Part print with two shaded views. Sizes in mm from the minimum x, y, z corner. Round coordinates to 2 decimals unless told otherwise and drop trailing zeros. Loops run counter-clockwise (first coordinate to the right, second up) from the corner with the lowest first, then second, coordinate; pieces in that order, holes last. Notation, with made-up numbers: (23.25, 9) -> (40.25, 9) arc R24 cw to (40.25, 22) -> close; hole circle Ø7 at (51.25, 21.25). An arc over 180 degrees is marked (long way). Use a Markdown table: item, result. Add a question column.
Item 1: Flat gauge pins, fed straight in: pin 1 (1.5 mm diameter, centred on x = 15, z = 4.5, fed in from -Y); pin 2 (1 mm diameter, centred on x = 18.5, z = 3, fed in from +Y); pin 3 (2 mm diameter, centred on x = 7.5, z = 10, fed in from +Y). Where does each tip first touch, or does it go through?
Item 2: Cut at A-A, the plane z = 12. List the corners of the cut face in (x, y).
Item 3: Cut at C-C, the plane x = 19. List the corners of the cut face in (y, z), plus the area to 3 significant figures.
Item 4: Cut at B-B, the plane y = 3.5. List the corners of the cut face in (x, z), plus the area to 3 significant figures.
Item 5: Probe line 1 (Y direction, x = 18, z = 1.75); line 2 (X direction, y = 9.5, z = 5) (1 decimal); line 3 (Y direction, x = 16, z = 8). List the from-to ranges inside material, lowest first. Write a range as [from, to].
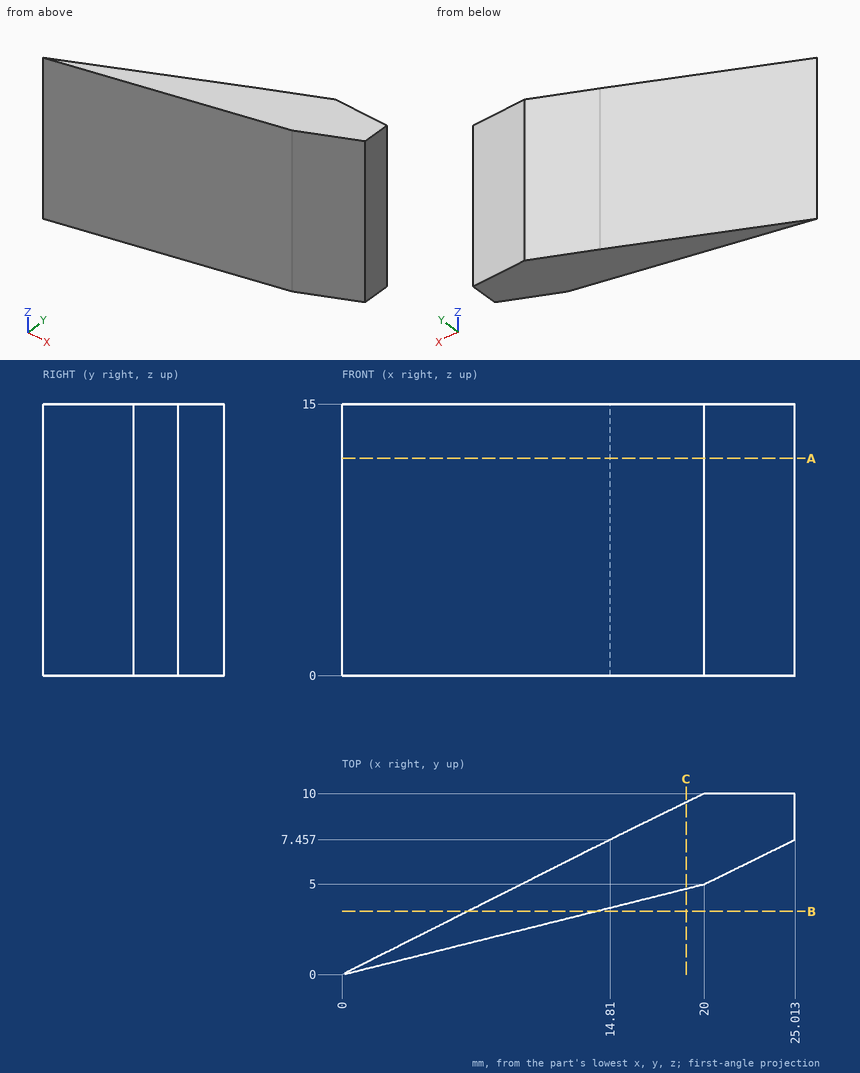
A:
| question | item | result |
|---|---|---|
| 1 | pin 1 | stops at y = 3.56 |
| 1 | pin 2 | stops at y = 9.51 |
| 1 | pin 3 | stops at y = 4.28 |
| 2 | outline | (0, 0) -> (20, 5) -> (25.01, 7.46) -> (25.01, 10) -> (20, 10) -> (14.81, 7.46) -> close |
| 3 | outline | (4.75, 0) -> (9.51, 0) -> (9.51, 15) -> (4.75, 15) -> close |
| 3 | area | 71.4 mm^2 |
| 4 | outline | (6.95, 0) -> (14, 0) -> (14, 15) -> (6.95, 15) -> close |
| 4 | area | 106 mm^2 |
| 5 | line 1 | y = [4.5, 9.02] |
| 5 | line 2 | x = [19, 25] |
| 5 | line 3 | y = [4, 8.04] |
